```python
from build123d import *

# Parameters (mm, degrees)
F0_R      = 5
F0_R_2    = 1.2
F1_DEPTH  = 0.5
F3_START  = 0.5
F3_DEPTH  = 6.8
F4_R      = 3
F5_DEPTH  = 0.5
F6_R      = 2.25
F6_R_2    = 2
F7_DEPTH  = 0.5
F9_DEPTH  = 17.751
F10_W     = 1.7
F10_H     = 14.5
F11_DEPTH = 25
F13_DEPTH = 14.5
F14_R     = 6
F15_DEPTH = 0.5


with BuildPart() as f1:
    # F0 (on Top) → F1 (new body)
    with BuildSketch(Plane.XY):
        with BuildLine():
            Line((0, 7.75), (-12.9, 7.75))
            Line((-12.9, 7.75), (-12.9, -7.75))
            Line((-12.9, -7.75), (0, -7.75))
            ThreePointArc((0, -7.75), (6.1399336055, -4.729029004), (7.4931417039, 1.978718627))
            ThreePointArc((7.4931417039, 1.978718627), (4.729029004, 6.1399336055), (0, 7.75))
        make_face()
        Circle(F0_R, mode=Mode.SUBTRACT)
        with BuildLine():
            ThreePointArc((7.4931417039, 1.978718627), (6.1399336055, -4.729029004), (0, -7.75))
            Line((0, -7.75), (7.1659829396, -9.9066614268))
            ThreePointArc((7.1659829396, -9.9066614268), (9.3288402344, -9.3819758335), (9.9270853869, -7.2382992285))
            Line((9.9270853869, -7.2382992285), (7.4931417039, 1.978718627))
        make_face()
        with Locations((7.8, -7.8)):
            Circle(F0_R_2, mode=Mode.SUBTRACT)
    extrude(amount=F1_DEPTH)

    # F2 (on Top) → F3 (join)
    with BuildSketch(Plane.XY.offset(F3_START)):
        with BuildLine():
            Line((-12.929528847, 7.75), (-12.929528847, -7.75))
            Line((-12.929528847, -7.75), (0, -7.75))
            ThreePointArc((0, -7.75), (7.75, 0), (0, 7.75))
            Line((0, 7.75), (-12.929528847, 7.75))
        make_face()
        with BuildLine():
            Line((-12.4, -7.25), (-12.4, 7.25))
            Line((-12.4, 7.25), (0, 7.25))
            ThreePointArc((0, 7.25), (7.25, 0), (0, -7.25))
            Line((0, -7.25), (-12.4, -7.25))
        make_face(mode=Mode.SUBTRACT)
    extrude(amount=F3_DEPTH)

    # F4 (on face) → F5 (cut, through all)
    with BuildSketch(Plane(origin=(0, 7.75, 0), x_dir=(-1, 0, 0), z_dir=(0, 1, 0))):
        with Locations((8.3, 3.65)):
            Circle(F4_R)
    extrude(amount=-F5_DEPTH, mode=Mode.SUBTRACT)

    # F6 (on face) → F7 (join)
    with BuildSketch(Plane(origin=(0, -7.25, 0), x_dir=(-1, 0, 0), z_dir=(0, 1, 0))):
        with Locations((8.3, 3.65)):
            Circle(F6_R)
        with Locations((8.3, 3.65)):
            Circle(F6_R_2, mode=Mode.SUBTRACT)
    extrude(amount=F7_DEPTH)

    # F8 (on face) → F9 (cut, through all)
    with BuildSketch(Plane(origin=(0, 7.75, 0), x_dir=(-1, 0, 0), z_dir=(0, 1, 0))):
        with BuildLine():
            Line((15.2742294595, 7.3), (8.3, 7.3))
            ThreePointArc((8.3, 7.3), (10.5687485064, 6.509244693), (11.8544696585, 4.479605597))
            Line((11.8544696585, 4.479605597), (12.9, 0))
            Line((12.9, 0), (15.2742294595, 7.3))
        make_face()
    extrude(amount=-F9_DEPTH, mode=Mode.SUBTRACT)

    # F10 (on face) → F11 (cut)
    with BuildSketch(Plane.XY.offset(0.5)):
        with Locations((-12.05, 0)):
            Rectangle(F10_W, F10_H)
    extrude(amount=F11_DEPTH, mode=Mode.SUBTRACT)

    # F12 (on face) → F13 (join, through all)
    with BuildSketch(Plane.XZ.offset(-7.25)):
        with BuildLine():
            Line((-8.3, 6.8), (-8.3, 7.3))
            ThreePointArc((-8.3, 7.3), (-10.5687485064, 6.509244693), (-11.8544696585, 4.479605597))
            Line((-11.8544696585, 4.479605597), (-12.7833010721, 0.5))
            Line((-12.7833010721, 0.5), (-12.4252442315, 0.5))
            Line((-12.4252442315, 0.5), (-11.3387916272, 4.479605597))
            ThreePointArc((-11.3387916272, 4.479605597), (-10.2117063542, 6.1535732095), (-8.3, 6.8))
        make_face()
    extrude(amount=F13_DEPTH)

    # F14 (on face) → F15 (join)
    with BuildSketch(Plane.XY.offset(7.3)):
        with BuildLine():
            Line((0, 7.25), (-8.3, 7.25))
            Line((-8.3, 7.25), (-8.3, -7.25))
            Line((-8.3, -7.25), (0, -7.25))
            ThreePointArc((0, -7.25), (7.25, 0), (0, 7.25))
        make_face()
        Circle(F14_R, mode=Mode.SUBTRACT)
    extrude(amount=-F15_DEPTH)


solid = f1.part
```
CAD build for the part. Positions are in the model's coordinates, mm. A direction names the side the tool comes from. Coordinates: 2 decimals unless noted, no trailing zeros. Write each loop counter-clockwise with the first axis right and the second up, starting at its lowest first coordinate (ties: lowest second). Pieces come first, ordered by that corner, then holes.
(1) Cut at B-B, the plane y = 6.75. List the corners of the cut face in (x, z), and give its area (3 significant figures).
(2) Cut at A-A, the plane x = 3.25. List the corners of the cut face in (y, z), and give its area (3 significant figures).
(3) Cut at D-D, the plane z = 3.65. List the corners of the cut face in (x, y), and give its area (3 significant figures).
(4) Flat gauge pins, fed straight in: pin 1 (1.3 mm diameter, centred on x = -9, z = 4.5, fed in from +Y); pin 2 (3 mm diameter, centred on x = 7.8, y = -7.8, fed in from +Z); pin 3 (4.5 mm diameter, centred on x = 0.5, y = 0.5, fed in from +Z); pin 4 (1 mm diameter, centred on y = 1.5, z = 2.5, fed in from -X). Where does each tip first touch, or does it go through?
(5) Two-plate mould, pull along X, no slides. Class faces 4 (the face through (8.727, -2.694, 0.246)), 5 (the face through (-6, 2, 7.3)), 6 (the face through (-11.89, 0.1, 2.46)): +X half, -X half, draft (parallel to the pull), parting line (faces both ways), or undercut.
(6) Drill centre lines: probe 1 along Z at (x, y) = (-8.3, -6.9); probe 2 along Z at (x, y) = (-5.5, 4); probe 3 along Y at (x, z) = (0, 0.4). Where is each one in solid material? Low to high.
(7) 3-axis set-ups, long thin cutter, end or side, ignore diameter. For faces 1 (the face through (-4, 7.25, 4)), 2 (the face through (-6, 0, 7)), 3 (the face through (-10.208, -7.004, 4.251)): which of +Z, -Z, +X, -X, +Y, -Y reach the whole face in a straight line?
(8) Cut at C-C, the plane y = -1.5. List the corners of the cut face in (x, z).
Geometry says:
1. outline: (-12.9, 0) - (3.81, 0) - (3.81, 7.3) - (-8.3, 7.3) arc R3.65 ccw to (-11.85, 4.48) - close; hole (-12.43, 0.5) - (2.65, 0.5) - (2.65, 6.8) - (-8.3, 6.8) arc R3.15 ccw to (-11.34, 4.48) - close
1. area: 25.7 mm2
2. outline: (-8.73, 0) - (-3.8, 0) - (-3.8, 0.5) - (-6.48, 0.5) - (-6.48, 6.8) - (-5.04, 6.8) - (-5.04, 7.3) - (-7.04, 7.3) - (-7.04, 0.5) - (-8.73, 0.5) - close; (3.8, 0) - (7.04, 0) - (7.04, 7.3) - (5.04, 7.3) - (5.04, 6.8) - (6.48, 6.8) - (6.48, 0.5) - (3.8, 0.5) - close
2. area: 13.1 mm2
3. outline: (-12.05, -7.75) - (0, -7.75) arc R7.75 ccw to (0, 7.75) - (-5.3, 7.75) - (-5.3, 7.25) - (0, 7.25) arc R7.25 cw to (0, -7.25) - (-6.05, -7.25) - (-6.05, -6.75) - (-6.3, -6.75) - (-6.3, -7.25) - (-10.3, -7.25) - (-10.3, -6.75) - (-10.55, -6.75) - (-10.55, -7.25) - (-11.57, -7.25) - (-11.57, 7.25) - (-11.3, 7.25) - (-11.3, 7.75) - (-12.05, 7.75) - close
3. area: 28.1 mm2
4. pin 1: stops at y = -7.25
4. pin 2: stops at z = 0.5
4. pin 3: passes through
4. pin 4: stops at x = -12.43
5. face 4: +X half
5. face 5: draft
5. face 6: undercut
6. probe 1: z = 0 to 0.5, 1.4 to 1.65, 5.65 to 5.9, 6.8 to 7.3
6. probe 2: z = 0 to 0.5, 6.8 to 7.3
6. probe 3: y = -7.75 to -5, 5 to 7.75
7. face 1: none
7. face 2: +Z
7. face 3: +Y
8. outline: (-12.9, 0) - (-4.77, 0) - (-4.77, 0.5) - (-12.43, 0.5) - (-11.34, 4.48) arc R3.15 cw to (-8.3, 6.8) - (-5.81, 6.8) - (-5.81, 7.3) - (-8.3, 7.3) arc R3.65 ccw to (-11.85, 4.48) - close; (4.77, 0) - (8.41, 0) - (8.41, 0.5) - (7.6, 0.5) - (7.6, 7.3) - (5.81, 7.3) - (5.81, 6.8) - (7.09, 6.8) - (7.09, 0.5) - (4.77, 0.5) - close
